from build123d import *

# Parameters (mm, degrees)
F1_DEPTH = 19
F2_T     = -4


with BuildPart() as f1:
    # F0 (on Front) → F1 (new body, symmetric)
    with BuildSketch(Plane.XZ):
        Polygon((-50, 25), (-50, -75), (50, -75), (50, 25), (19, 50), (19, 90), (-19, 90), (-19, 50), align=None)
    extrude(amount=F1_DEPTH, both=True)

    # F2
    f2_openings = [f1.faces().sort_by_distance(p)[0] for p in [
        (0, -19, -6.201711),
    ]]
    offset(amount=F2_T, openings=f2_openings, kind=Kind.INTERSECTION)


solid = f1.part
Geometry check sheet. Reference: the model listing, model coordinates, mm. A direction names the side the tool comes from. Coordinates: 2 decimals unless noted, no trailing zeros. Order: outer loops, then holes, each group sorted by start corner. A loop starts at its lowest first (then second) coordinate and runs counter-clockwise, first axis right, second up. Notation, with made-up numbers: (6.5, -12) - (15.5, -12) arc R12 ccw to (15.5, -5) - close; hole circle Ø8 at (80, -38). An arc over 180 degrees is marked (long way). Answer in a Markdown table with one row per item. Add a question column.
1) Release check for a two-part mould opening along Z. For faces 6 (the flat face through (-1, -2, -71)), 7 (the flat face through (-1, 15, -9)), 8 (the flat face through (34.717, -0.266, 37.325)), 9 (the flat face through (50, 0, -26)) record: +Z half, -Z half, draft (parallel to the pull), parting line (faces both ways), or undercut.
2) Gauge pin test, flat ends, axial feed: P1, Ø17, axis at y = -3, z = 76.5, coming from the -X side; P2, Ø2, axis at x = -31.5, z = -54.5, coming from the -Y side; P3, Ø17, axis at y = 6, z = 75, coming from the +X side. Record the tip position at first contact, or that the pin passes through.
3) Cross-section at B-B, the plane z = -3.5. Record the cut outline in (x, y), then the cut area to 3 significant figures.
4) Material ranges on line 1 along Z through (x, y) = (-8.5, 1); line 2 along X through (y, z) = (13, 7); line 3 along Y through (x, z) = (-33, -43.5), recorded low to high. Write a range as [from, to].
5) Set-up check for faces 1 (the flat face through (-48, -19, 2)), 2 (the flat face through (-46, -2, -23)), 3 (the flat face through (-1, 19, -10)), 4 (the flat face through (19, 0, 70)), 5 (the flat face through (-19, 0, 70)): record each of +Z, -Z, +X, -X, +Y, -Y from which the full face is reachable in a straight line by a thin tool's end or side.
6) Cross-section at C-C, the plane x = -4.5. Record the cut outline in (y, z).
7) Cross-section at A-A, the plane y = -5.5. Record the cut outline in (x, z).
Check result:
| question | item | result |
|---|---|---|
| 1 | face 6 | undercut |
| 1 | face 7 | undercut |
| 1 | face 8 | +Z half |
| 1 | face 9 | draft |
| 2 | P1 | stops at x = -19 |
| 2 | P2 | stops at y = 15 |
| 2 | P3 | stops at x = 19 |
| 3 | outline | (-50, -19) - (-46, -19) - (-46, 15) - (46, 15) - (46, -19) - (50, -19) - (50, 19) - (-50, 19) - close |
| 3 | area | 672 mm² |
| 4 | line 1 | z = [-75, -71], [86, 90] |
| 4 | line 2 | x = [-50, -46], [46, 50] |
| 4 | line 3 | y = [15, 19] |
| 5 | face 1 | +Z, -Z, +X, -X, -Y |
| 5 | face 2 | -Y |
| 5 | face 3 | +Z, -Z, +X, -X, +Y |
| 5 | face 4 | +Z, +X, +Y, -Y |
| 5 | face 5 | +Z, -X, +Y, -Y |
| 6 | outline | (-19, -75) - (19, -75) - (19, 90) - (-19, 90) - (-19, 86) - (15, 86) - (15, -71) - (-19, -71) - close |
| 7 | outline | (-50, -75) - (50, -75) - (50, 25) - (19, 50) - (19, 90) - (-19, 90) - (-19, 50) - (-50, 25) - close; hole (-46, -71) - (46, -71) - (46, 23.09) - (15, 48.09) - (15, 86) - (-15, 86) - (-15, 48.09) - (-46, 23.09) - close |
